from build123d import *

# Parameters (mm, degrees)
BOSS_EXTRUDE1_DEPTH               = 4.5
M5_CLEARANCE_HOLE1_D              = 5.5
M5_CLEARANCE_HOLE1_CSINK_D        = 5.55
M5_CLEARANCE_HOLE1_CSINK_ANGLE    = 90
SKETCH5_R                         = 12.5
CUT_EXTRUDE1_DEPTH                = 81.825429167
SKETCH12_W                        = 45
SKETCH12_H                        = 24.5
BOSS_EXTRUDE2_DEPTH               = 4.5
F_1_4_CLEARANCE_HOLE1_D           = 7.14248
F_1_4_CLEARANCE_HOLE1_CSINK_D     = 8.41248
F_1_4_CLEARANCE_HOLE1_CSINK_ANGLE = 90
FILLET1_R                         = 10
FILLET2_R                         = 2
SKETCH18_W                        = 106.323058396
SKETCH18_H                        = 71.002809098
CUT_EXTRUDE4_DEPTH                = 60
M4_CLEARANCE_HOLE1_D              = 4.8
BOSS_EXTRUDE3_DEPTH               = 4.5
FILLET3_R                         = 10
FILLET3_OF_MIRROR1_R              = 10


with BuildPart() as part:
    # Sketch1 → Boss-Extrude1 (new body)
    with BuildSketch(Plane(origin=(0, 0, 0), x_dir=(1, 0, 0), z_dir=(0, 1, 0))):
        with BuildLine():
            Line((-22.5, -77.5), (22.5, -77.5))
            Line((22.5, -77.5), (22.5, 3.34e-07))
            ThreePointArc((22.5, 3.34e-07), (0, 22.5), (-22.5, 3.34e-07))
            Line((-22.5, 3.34e-07), (-22.5, -77.5))
        make_face()
    extrude(amount=BOSS_EXTRUDE1_DEPTH)

    # M5 Clearance Hole1 (through all)
    with Locations(Plane(origin=(0, 4.5, 0), x_dir=(1, 0, 0), z_dir=(0, 1, 0))):
        with Locations((-6.696960066, -16.167891819), (6.696960066, -16.167891819), (6.696960066, 16.167891819), (-6.696960066, 16.167891819)):
            CounterSinkHole(M5_CLEARANCE_HOLE1_D / 2, M5_CLEARANCE_HOLE1_CSINK_D / 2, counter_sink_angle=M5_CLEARANCE_HOLE1_CSINK_ANGLE)

    # Sketch5 → Cut-Extrude1 (cut, through all)
    with BuildSketch(Plane(origin=(0, 4.5, 0), x_dir=(1, 0, 0), z_dir=(0, 1, 0))):
        with Locations(Location((0, 0, 0), (0, 0, 270))):
            Circle(SKETCH5_R)
    extrude(amount=-CUT_EXTRUDE1_DEPTH, mode=Mode.SUBTRACT)

    # Sketch12 → Boss-Extrude2 (add)
    with BuildSketch(Plane.XY.offset(77.5)):
        with Locations((0, 12.25)):
            Rectangle(SKETCH12_W, SKETCH12_H)
    extrude(amount=BOSS_EXTRUDE2_DEPTH)

    # 1/4 Clearance Hole1 (through all)
    with Locations(Plane(origin=(0, 0, 77.5), x_dir=(-1, 0, 0), z_dir=(0, 0, -1))):
        with Locations((0, 14.5)):
            CounterSinkHole(F_1_4_CLEARANCE_HOLE1_D / 2, F_1_4_CLEARANCE_HOLE1_CSINK_D / 2, counter_sink_angle=F_1_4_CLEARANCE_HOLE1_CSINK_ANGLE)

    # Fillet1
    fillet1_edges = [part.edges().sort_by_distance(p)[0] for p in [
        (22.5, 24.5, 79.75),
        (-22.5, 24.5, 79.75),
    ]]
    fillet(fillet1_edges, radius=FILLET1_R)

    # Fillet2
    fillet2_edges = [part.edges().sort_by_distance(p)[0] for p in [
        (0, 4.5, 77.5),
        (0, 0, 82),
    ]]
    fillet(fillet2_edges, radius=FILLET2_R)

    # Sketch18 → Cut-Extrude4 (cut)
    with BuildSketch(Plane.XY.offset(-22.5)):
        with Locations((20.664180994, 31.016391908)):
            Rectangle(SKETCH18_W, SKETCH18_H)
    extrude(amount=CUT_EXTRUDE4_DEPTH, mode=Mode.SUBTRACT)

    # M4 Clearance Hole1 (through all)
    with Locations(Plane(origin=(0, 0, 0), x_dir=(-1, 0, 0), z_dir=(0, -1, 0))):
        with Locations((10.58478565, -44.5), (-10.58478565, -44.5)):
            Hole(M4_CLEARANCE_HOLE1_D / 2)

    # Sketch23 → Boss-Extrude3 (add)
    with BuildSketch(Plane.ZY.offset(22.5)):
        Polygon((77.5, 14.5), (57.5, 4.5), (77.5, 4.5), align=None)
    boss_extrude3 = extrude(amount=-BOSS_EXTRUDE3_DEPTH)

    # Fillet3
    fillet3_edges = [part.edges().sort_by_distance(p)[0] for p in [
        (-20.25, 14.5, 77.5),
        (-20.25, 4.5, 57.5),
    ]]
    fillet(fillet3_edges, radius=FILLET3_R)

    # Mirror1: Boss-Extrude3 across plane
    add(boss_extrude3.mirror(Plane(origin=(0, 0, 0), x_dir=(0, 0, 1), z_dir=(1, 0, 0))))

    # Fillet3 of Mirror1
    fillet3_of_mirror1_edges = [part.edges().sort_by_distance(p)[0] for p in [
        (20.25, 14.5, 77.5),
        (20.25, 4.5, 57.5),
    ]]
    fillet(fillet3_of_mirror1_edges, radius=FILLET3_OF_MIRROR1_R)


solid = part.part
Here's how the part is built. I have some questions about the finished solid (model axes, mm). A direction names the side the tool comes from. Coordinates: 2 decimals unless noted, no trailing zeros. Order: outer loops, then holes, each group sorted by start corner. A loop starts at its lowest first (then second) coordinate and runs counter-clockwise, first axis right, second up. Notation, with made-up numbers: (29.5, 85.25) - (55.5, 85.25) arc R27 cw to (55.5, 123.25) - close; hole circle Ø11 at (-25.75, 33.5). An arc over 180 degrees is marked (long way). Use CSV: the item, a comma, the result in double quotes. Start each with the question number.
1. I'm going to push flat-ended pins straight in: pin 1 (4 mm diameter, centred on x = -7.5, y = 21.5, fed in from -Z); pin 2 (19 mm diameter, centred on x = 0.5, z = 56, fed in from +Y). Where does each tip first touch, or does it pass through?
2. If we mould it in two halves opening along Y, with no side actions, what happens to faces 3 (the face through (10.06, 2.28, 46.84)), 4 (the face through (0, 4.5, 56)), 5 (the face through (0, 0, 58))? For each: +Y half, -Y half, draft (parallel to the pull), parting line (faces both ways), or undercut.
3. Suppose I cut it at A-A on x = 0. List the corners of the cut face in (y, z) for me (3 decimals), then the cut area to 3 significant figures.
4. Suppose I cut it at B-B on z = 44.5. List the corners of the cut face in (x, y) for me.
5. For faces 1 (the face through (18, 8, 71)), 2 (the face through (-9.48, 2.28, 46.63)), which set-ups out of +Z, -Z, +X, -X, +Y, -Y let a thin tool reach every point of the face, with its end or its side?
6. Suppose I cut it at C-C on z = 79. List the corners of the cut face in (x, y) for me, then the cut area to 3 significant figures.
7. Please list where these lines run through material, in increasing order: line 1 (X direction, y = 2.35, z = 44.5); line 2 (Y direction, x = 0, z = 80); line 3 (X direction, y = 14.5, z = 79.9). Write a range as from..to.
8. Suppose I cut it at D-D on x = 5. List the corners of the cut face in (y, z) for me, then the cut area to 3 significant figures.
Output:
1,pin 1,"stops at z = 77.5"
1,pin 2,"stops at y = 4.5"
2,face 3,"draft"
2,face 4,"+Y half"
2,face 5,"-Y half"
3,outline,"(0, 37.5) - (4.5, 37.5) - (4.5, 75.5) arc R2 cw to (6.5, 77.5) - (10.294, 77.5) - (10.929, 78.135) - (10.929, 82) - (2, 82) arc R2 ccw to (0, 80) - close; (18.071, 78.135) - (18.706, 77.5) - (24.5, 77.5) - (24.5, 82) - (18.071, 82) - close"
3,area,"258 mm2"
4,outline,"(-22.5, 0) - (-12.98, 0) - (-12.98, 4.5) - (-22.5, 4.5) - close; (-8.18, 0) - (8.18, 0) - (8.18, 4.5) - (-8.18, 4.5) - close; (12.98, 0) - (22.5, 0) - (22.5, 4.5) - (12.98, 4.5) - close"
5,face 1,"-Z, +Y"
5,face 2,"+Y, -Y"
6,outline,"(-22.5, 0) - (22.5, 0) - (22.5, 14.5) arc R10 ccw to (12.5, 24.5) - (-12.5, 24.5) arc R10 ccw to (-22.5, 14.5) - close; hole circle Ø7.14 at (0, 14.5)"
6,area,"1,020 mm2"
7,line 1,"x = -22.5..-12.98, -8.18..8.18, 12.98..22.5"
7,line 2,"y = 0..10.93, 18.07..24.5"
7,line 3,"x = -22.5..-3.57, 3.57..22.5"
8,outline,"(0, 37.5) - (4.5, 37.5) - (4.5, 75.5) arc R2 cw to (6.5, 77.5) - (24.5, 77.5) - (24.5, 82) - (2, 82) arc R2 ccw to (0, 80) - close"
8,area,"290 mm2"
